from build123d import *

# Parameters (mm, degrees)
SKETCH1_R                       = 81.15
SKETCH1_R_2                     = 77.15
BOSS_EXTRUDE1_DEPTH             = 12.5
SKETCH2_W                       = 5
SKETCH2_H                       = 5
CUT_EXTRUDE2_DEPTH              = 116.44217167
CIRPATTERN1_COUNT               = 16
CIRPATTERN1_ANGLE               = 168.75
CIRPATTERN1_THE_OTHER_WAY_COUNT = 16
CIRPATTERN1_THE_OTHER_WAY_ANGLE = 168.75
BOSS_EXTRUDE2_DEPTH             = 1
BOSS_EXTRUDE2_DEPTH_BACK        = 13.5


with BuildPart() as part:
    # Sketch1 → Boss-Extrude1 (new body)
    with BuildSketch(Plane(origin=(0, 0, 0), x_dir=(1, 0, 0), z_dir=(0, 1, 0))):
        with Locations(Location((0, 0, 0), (0, 0, 270))):
            Circle(SKETCH1_R)
        with Locations(Location((0, 0, 0), (0, 0, 270))):
            Circle(SKETCH1_R_2, mode=Mode.SUBTRACT)
    extrude(amount=BOSS_EXTRUDE1_DEPTH)

    # Sketch2 → Cut-Extrude2 (cut, through all)
    with BuildSketch(Plane.XY):
        with Locations((0, 6.25)):
            Rectangle(SKETCH2_W, SKETCH2_H)
    cut_extrude2 = extrude(amount=-CUT_EXTRUDE2_DEPTH, mode=Mode.SUBTRACT)

    # CirPattern1: Cut-Extrude2 ×16 about axis
    cirpattern1_axis = Axis((0, 0, 0), (0, 1, 0))
    for i in range(1, CIRPATTERN1_COUNT):
        add(cut_extrude2.rotate(cirpattern1_axis, i * CIRPATTERN1_ANGLE / (CIRPATTERN1_COUNT - 1)), mode=Mode.SUBTRACT)

    # CirPattern1 the other way: Cut-Extrude2 ×16 about axis
    cirpattern1_the_other_way_axis = Axis((0, 0, 0), (0, -1, 0))
    for i in range(1, CIRPATTERN1_THE_OTHER_WAY_COUNT):
        add(cut_extrude2.rotate(cirpattern1_the_other_way_axis, i * CIRPATTERN1_THE_OTHER_WAY_ANGLE / (CIRPATTERN1_THE_OTHER_WAY_COUNT - 1)), mode=Mode.SUBTRACT)

    # Sketch3 → Boss-Extrude2 (add, two sides: drawn at the far end of the back side and taken through both)
    with BuildSketch(Plane(origin=(0, 12.5, 0), x_dir=(1, 0, 0), z_dir=(0, 1, 0)).offset(-BOSS_EXTRUDE2_DEPTH_BACK)):
        with BuildLine():
            Line((-10.515914532, -75.420408654), (-11.372101927, -81.561006601))
            ThreePointArc((-11.372101927, -81.561006601), (-0.879882913, -82.345299235), (9.626699335, -81.785384757))
            Line((9.626699335, -81.785384757), (8.901920515, -75.627893737))
            ThreePointArc((8.901920515, -75.627893737), (-0.813637934, -76.145653148), (-10.515914532, -75.420408654))
        make_face()
    extrude(amount=BOSS_EXTRUDE2_DEPTH + BOSS_EXTRUDE2_DEPTH_BACK)


solid = part.part
The listing builds one solid part. Answer for the finished solid, in the listing's coordinates (mm). A direction names the side the tool comes from. Round coordinates to 2 decimals unless told otherwise and drop trailing zeros. Order: outer loops, then holes, each group sorted by start corner. A loop starts at its lowest first (then second) coordinate and runs counter-clockwise, first axis right, second up. Notation, with made-up numbers: M 29.5,8 L 56.5,8 A15 cw 56.5,19 Z; hole C -23.5,47.25 d7. An arc over 180 degrees is marked long. Answer in a Markdown table with one row per item. Add a question column.
1) The part is cut by section A-A on z = 0. Determine the outline of the cut face in (x, y).
2) Consider line 1 along X through (y, z) = (3.5, 0); line 2 along Z through (x, y) = (0, 9.75); line 3 along Y through (x, z) = (-33, -73). Determine where each line is inside the solid, lowest interval first. Write a range as from..to.
3) The part is cut by section B-B on x = 0. Determine the outline of the cut face in (y, z), plus the area to 3 significant figures.
4) Which of the six approach directions +Z, -Z, +X, -X, +Y, -Y give full straight-line access (tool end or side, diameter ignored) to faces 1 (the face through (-1, 13.5, 79)), 2 (the face through (-77.08, 6.22, -17.88)), 3 (the face through (-66, 8.75, 44)), 4 (the face through (-79, 6, -2.5))?
5) Determine the mould class of faces 5 (the face through (-2.5, 6, -79)), 6 (the face through (-32.573, 6.215, -72.106)), 7 (the face through (-27.954, 6.215, 74.019)) for opening direction Z: pulls with the +Z half, pulls with the -Z half, needs draft (parallel to the pull), parting line crosses it, or undercut.
6) Flat-ended cylindrical pins translate along their axes: pin 1 Ø6 at (x, z) = (-72, 29.5) entering from -Y; pin 2 Ø2.5 at (x, z) = (77, 17) entering from +Y; pin 3 Ø1.5 at (x, y) = (-48.5, 3.5) entering from -Z. Find the tip coordinate at first contact, or state that the pin passes through.
7) The part is cut by section C-C on z = 25. Determine the outline of the cut face in (x, y), plus the area to 3 significant figures.
Findings below:
| question | item | result |
|---|---|---|
| 1 | outline | M -81.15,0 L -77.15,0 L -77.15,3.75 L -81.15,3.75 Z; M -81.15,8.75 L -77.15,8.75 L -77.15,12.5 L -81.15,12.5 Z; M 77.15,0 L 81.15,0 L 81.15,3.75 L 77.15,3.75 Z; M 77.15,8.75 L 81.15,8.75 L 81.15,12.5 L 77.15,12.5 Z |
| 2 | line 1 | x = -81.15..-77.15, 77.15..81.15 |
| 2 | line 2 | z = -81.15..-77.15, 76.15..82.35 |
| 2 | line 3 | y = 0..12.5 |
| 3 | outline | M -1,76.15 L 13.5,76.15 L 13.5,82.35 L -1,82.35 Z; M 0,-81.15 L 3.75,-81.15 L 3.75,-77.15 L 0,-77.15 Z; M 8.75,-81.15 L 12.5,-81.15 L 12.5,-77.15 L 8.75,-77.15 Z |
| 3 | area | 120 mm² |
| 4 | face 1 | +Z, -Z, +X, -X, +Y |
| 4 | face 2 | -X |
| 4 | face 3 | none |
| 4 | face 4 | +X, -X |
| 5 | face 5 | needs draft |
| 5 | face 6 | pulls with the -Z half |
| 5 | face 7 | undercut |
| 6 | pin 1 | stops at y = 0 |
| 6 | pin 2 | stops at y = 12.5 |
| 6 | pin 3 | stops at z = -65.61 |
| 7 | outline | M -77.2,0 L -72.99,0 L -72.99,12.5 L -77.2,12.5 Z; M 72.99,0 L 77.2,0 L 77.2,12.5 L 72.99,12.5 Z |
| 7 | area | 105 mm² |
